from build123d import *

# Parameters (mm, degrees)
F2_W     = 603
F2_H     = 535
F2_R     = 10
F2_R_2   = 201
F3_DEPTH = 3
F4_W     = 3
F4_H     = 535
F4_W_2   = 487
F4_H_2   = 3
F5_DEPTH = 50
F6_R     = 13
F6_R_2   = 10
F7_DEPTH = 50


with BuildPart() as f1:
    # F0 (on Front) → F1 (revolve)
    with BuildSketch(Plane.XZ):
        Polygon((-250, 3), (-200, 3), (-200, 55), (-201, 55), (-201, 95), (-249, 95), (-249, 55), (-250, 55), align=None)
        Polygon((-10, 3), (-200, 3), (-250, 3), (-250, 0), (-10, 0), align=None)
    revolve(axis=Axis((0, 0, 187.921241), (0, 0, -1)))

    # F2 (on Top) → F3 (join)
    with BuildSketch(Plane.XY):
        Rectangle(F2_W, F2_H)
        with Locations((-271.5, -237.5)):
            Circle(F2_R, mode=Mode.SUBTRACT)
        with Locations((271.5, -237.5)):
            Circle(F2_R, mode=Mode.SUBTRACT)
        with Locations((-271.5, 237.5)):
            Circle(F2_R, mode=Mode.SUBTRACT)
        Circle(F2_R_2, mode=Mode.SUBTRACT)
        with Locations((271.5, 237.5)):
            Circle(F2_R, mode=Mode.SUBTRACT)
    extrude(amount=F3_DEPTH)

    # F4 (on face) → F5 (join)
    with BuildSketch(Plane.XY.offset(3)):
        with Locations((-300, 0)):
            Rectangle(F4_W, F4_H)
        with Locations((300, 0)):
            Rectangle(F4_W, F4_H)
        with Locations((0, -266)):
            Rectangle(F4_W_2, F4_H_2)
        with Locations((0, 266)):
            Rectangle(F4_W_2, F4_H_2)
    extrude(amount=-F5_DEPTH)

    # F6 (on face) → F7 (join)
    with BuildSketch(Plane(origin=(0, 0, 0), x_dir=(1, 0, 0), z_dir=(0, 0, -1))):
        Circle(F6_R)
        Circle(F6_R_2, mode=Mode.SUBTRACT)
    extrude(amount=F7_DEPTH)


solid = f1.part
Geometry: final body of the model. Coordinates: model frame, mm. A direction names the side the tool comes from. Round coordinates to 2 decimals unless told otherwise and drop trailing zeros. Order: outer loops, then holes, each group sorted by start corner. A loop starts at its lowest first (then second) coordinate and runs counter-clockwise, first axis right, second up.
Q1. Section D-D, the plane x = 271.5. Output: boundary loops of the cut face in (y, z).
Result sheet:
outline: (-267.5, 0) - (-247.5, 0) - (-247.5, 3) - (-267.5, 3) - close; (-227.5, 0) - (227.5, 0) - (227.5, 3) - (-227.5, 3) - close; (247.5, 0) - (267.5, 0) - (267.5, 3) - (247.5, 3) - close
Q2. Pin query (flat end, axial travel): pin 1 (12 mm diameter, centred on x = -71, y = 128, fed in from +Z); pin 2 (18 mm diameter, centred on x = 271.5, y = -237.5, fed in from +Z); pin 3 (3.5 mm diameter, centred on x = -300, y = 90, fed in from -Z); pin 4 (1.5 mm diameter, centred on y = 75, z = 29, fed in from +X). Return the tip coordinate at first contact, or that it passes through.
Result sheet:
pin 1: stops at z = 3
pin 2: passes through
pin 3: stops at z = -47
pin 4: stops at x = 238.72
Q3. Mould query, pull axis Y, two halves, no side actions, for faces 1 (the face through (-3, -42, 3)), 2 (the face through (301.5, -4, -22)), 3 (the face through (-4, 267.5, -22)). Classes: released by +Y, released by -Y, zero draft, split by the parting line, or undercut.
Result sheet:
face 1: undercut
face 2: zero draft
face 3: released by +Y
Q4. Material intervals for probe 1 along Y at (x, z) = (0, -30); probe 2 along Y at (x, z) = (-271.5, 1.65); probe 3 along Y at (x, z) = (0, 1.3), sorted ascending.
Result sheet:
probe 1: y = -267.5 to -264.5, -13 to -10, 10 to 13, 264.5 to 267.5
probe 2: y = -267.5 to -247.5, -227.5 to 227.5, 247.5 to 267.5
probe 3: y = -267.5 to -10, 10 to 267.5
Q5. Access query for faces 4 (the face through (-180, -177, 3)), 5 (the face through (-3, -264.5, -23)), 6 (the face through (298.5, -4, -23)). Directions: +Z, -Z, +X, -X, +Y, -Y. A direction counts if a zero-diameter tool reaches every point of the face in a straight line with its end or side. Return the directions, or none.
Result sheet:
face 4: +Z
face 5: -Z
face 6: -Z, +Y, -Y
Q6. Section A-A, the plane z = -8. Output: boundary loops of the cut face in (x, y).
Result sheet:
outline: (-301.5, -267.5) - (-298.5, -267.5) - (-298.5, 267.5) - (-301.5, 267.5) - close; (-243.5, -267.5) - (243.5, -267.5) - (243.5, -264.5) - (-243.5, -264.5) - close; (-243.5, 264.5) - (243.5, 264.5) - (243.5, 267.5) - (-243.5, 267.5) - close; circle Ø26 at (0, 0); (298.5, -267.5) - (301.5, -267.5) - (301.5, 267.5) - (298.5, 267.5) - close; hole circle Ø20 at (0, 0)
